Check sheet for the modelled part. Datum: model origin and axes. Units: mm. Face numbers are marked on the shaded views. A direction names the side the tool comes from. Coordinates: 2 decimals unless noted, no trailing zeros. Loops run counter-clockwise (first coordinate to the right, second up) from the corner with the lowest first, then second, coordinate; pieces in that order, holes last.
```python
from build123d import *

# Parameters (mm, degrees)
SKETCH2_W           = 6
SKETCH2_H           = 18
BOSS_EXTRUDE1_DEPTH = 6
SKETCH3_R           = 2.25
CUT_EXTRUDE1_DEPTH  = 12.22497216
SKETCH4_W           = 4.5
SKETCH4_H           = 12
CUT_EXTRUDE2_DEPTH  = 13.369316877


with BuildPart() as part:
    # Sketch2 → Boss-Extrude1 (new body)
    with BuildSketch(Plane.XY):
        Rectangle(SKETCH2_W, SKETCH2_H)
    extrude(amount=BOSS_EXTRUDE1_DEPTH)

    # Sketch3 → Cut-Extrude1 (cut, through all)
    with BuildSketch(Plane.XY.offset(6)):
        with Locations((0, -6)):
            Circle(SKETCH3_R)
    extrude(amount=-CUT_EXTRUDE1_DEPTH, mode=Mode.SUBTRACT)

    # Sketch4 → Cut-Extrude2 (cut, through all)
    with BuildSketch(Plane(origin=(3, 0, 0), x_dir=(0, 0, -1), z_dir=(1, 0, 0))):
        with Locations((-3, 3)):
            Rectangle(SKETCH4_W, SKETCH4_H)
    extrude(amount=-CUT_EXTRUDE2_DEPTH, mode=Mode.SUBTRACT)


solid = part.part
```
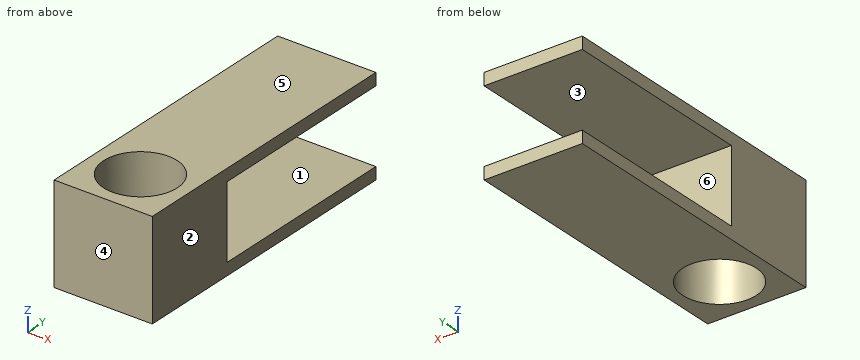
1) Scan lines: line 1 (Z direction, x = 2.05, y = 4.25); line 2 (Y direction, x = 0, z = 2.45); line 3 (Y direction, x = -2.05, z = 4.6). Record each from-to range of solid material in increasing order.
Answer sheet:
line 1: z = 0 to 0.75, 5.25 to 6
line 2: y = -9 to -8.25, -3.75 to -3
line 3: y = -9 to -6.93, -5.07 to -3
2) Depth check by flat-ended pin: pin 1 (2 mm diameter, centred on x = 0, z = 3.5, fed in from +Y). Enter the tip coordinate at first touch or a pass-through.
Answer sheet:
pin 1: stops at y = -3
3) Set-up check for the marked faces 1 and 2: record each of +Z, -Z, +X, -X, +Y, -Y from which the full face is reachable in a straight line by a thin tool's end or side.
Answer sheet:
face 1: +X, -X, +Y
face 2: +Z, -Z, +X, +Y, -Y
4) Section check A-A on x = 0. Enter the section's corners in (y, z), plus the area to 3 significant figures.
Answer sheet:
outline: (-9, 0) - (-8.25, 0) - (-8.25, 6) - (-9, 6) - close; (-3.75, 0) - (9, 0) - (9, 0.75) - (-3, 0.75) - (-3, 5.25) - (9, 5.25) - (9, 6) - (-3.75, 6) - close
area: 27.0 mm2
5) Mould release check, pull along Z, two halves, no side actions. Record for the marked faces 3, 4, 5 and 6: +Z half, -Z half, draft (parallel to the pull), parting line (faces both ways), or undercut.
Answer sheet:
face 3: undercut
face 4: draft
face 5: +Z half
face 6: undercut
6) Section check D-D on z = 2.45. Enter the section's corners in (x, y).
Answer sheet:
outline: (-3, -9) - (3, -9) - (3, -3) - (-3, -3) - close; hole circle Ø4.5 at (0, -6)
7) Section check C-C on z = 5.45. Enter the section's corners in (x, y), plus the area to 3 significant figures.
Answer sheet:
outline: (-3, -9) - (3, -9) - (3, 9) - (-3, 9) - close; hole circle Ø4.5 at (0, -6)
area: 92.1 mm2
8) Section check B-B on y = -6. Enter the section's corners in (x, z).
Answer sheet:
outline: (-3, 0) - (-2.25, 0) - (-2.25, 6) - (-3, 6) - close; (2.25, 0) - (3, 0) - (3, 6) - (2.25, 6) - close
